Can you work these out from the model? Positions are in its coordinate system, mm. Coordinates: 2 decimals unless noted, no trailing zeros. Loops run counter-clockwise (first coordinate to the right, second up) from the corner with the lowest first, then second, coordinate; pieces in that order, holes last. Notation, with made-up numbers: (29.5, 64) -> (50.5, 64) arc R25 ccw to (50.5, 86) -> close; hole circle Ø10 at (74.5, 65). An arc over 180 degrees is marked (long way). Put each result on its own line as item: value. Start each with the question number.
Item 1: Will this pin go through, and if not, where does the flat tip stop? P1, Ø2.5, axis at x = -91.5, y = -22.5, coming from the +Z side.
Item 2: If we section it at A-A on y = 0: Please give me the cut outline in (x, z), plus the area to 3 significant figures.
Item 3: We'd pull the mould along X, two halves only. Please class faces 1 (the flat face through (-1, 1, 0)), 2 (the cylindrical face through (12.1, -1.2, 1.5)), 3 (the cylindrical face through (-103.08, 35.16, 1.52)): pulls with the +X half, pulls with the -X half, needs draft (parallel to the pull), parting line crosses it, or undercut.
Item 4: Please list where these lines run through material, in increasing order: L1, parallel to Y at x = 102.5, z = 0.85; L2, parallel to Y at x = 10.5, z = 2; L3, parallel to X at y = 1.5, z = 1.6. Write a range as from..to.
```python
from build123d import *

# Parameters (mm, degrees)
SKETCH1_W           = 213
SKETCH1_H           = 77.54
BOSS_EXTRUDE1_DEPTH = 3
FILLET2_R           = 12
CUT_EXTRUDE1_REACH  = 115.377
SKETCH2_R           = 2
CUT_EXTRUDE2_REACH  = 115.377
SKETCH3_R           = 1.5
CUT_EXTRUDE3_REACH  = 115.377
SKETCH4_R           = 1.5


with BuildPart() as part:
    # Sketch1 → Boss-Extrude1 (new body)
    with BuildSketch(Plane.XY):
        Rectangle(SKETCH1_W, SKETCH1_H)
    extrude(amount=BOSS_EXTRUDE1_DEPTH)

    # Fillet2
    fillet2_edges = [part.edges().sort_by_distance(p)[0] for p in [
        (-106.5, 38.77, 1.5),
    ]]
    fillet(fillet2_edges, radius=FILLET2_R)

    # Sketch2 → Cut-Extrude1 (cut, up to next)
    with BuildSketch(Plane(origin=(0, 0, 0), x_dir=(-1, 0, 0), z_dir=(0, 0, -1)), mode=Mode.PRIVATE) as cut_extrude1_sk1:
        with Locations((-10.5, 0)):
            Circle(SKETCH2_R)
    cut_extrude1_tool1 = extrude(cut_extrude1_sk1.sketch, amount=-CUT_EXTRUDE1_REACH, mode=Mode.PRIVATE) & part.part
    add(cut_extrude1_tool1.solids().sort_by_distance((10.5, 0, 0))[0], mode=Mode.SUBTRACT)

    # Sketch3 → Cut-Extrude2 (cut, up to next)
    with BuildSketch(Plane(origin=(0, 0, 0), x_dir=(-1, 0, 0), z_dir=(0, 0, -1)), mode=Mode.PRIVATE) as cut_extrude2_sk1:
        with Locations((-102.5, 22.5)):
            Circle(SKETCH3_R)
    cut_extrude2_tool1 = extrude(cut_extrude2_sk1.sketch, amount=-CUT_EXTRUDE2_REACH, mode=Mode.PRIVATE) & part.part
    # Sketch3 → Cut-Extrude2 (cut, up to next)
    with BuildSketch(Plane(origin=(0, 0, 0), x_dir=(-1, 0, 0), z_dir=(0, 0, -1)), mode=Mode.PRIVATE) as cut_extrude2_sk2:
        with Locations((-102.5, -22.5)):
            Circle(SKETCH3_R)
    cut_extrude2_tool2 = extrude(cut_extrude2_sk2.sketch, amount=-CUT_EXTRUDE2_REACH, mode=Mode.PRIVATE) & part.part
    add(cut_extrude2_tool1.solids().sort_by_distance((102.5, 22.5, 0))[0], mode=Mode.SUBTRACT)
    add(cut_extrude2_tool2.solids().sort_by_distance((102.5, -22.5, 0))[0], mode=Mode.SUBTRACT)

    # Sketch4 → Cut-Extrude3 (cut, up to next)
    with BuildSketch(Plane(origin=(0, 0, 0), x_dir=(-1, 0, 0), z_dir=(0, 0, -1)), mode=Mode.PRIVATE) as cut_extrude3_sk1:
        with Locations((91.5, 22.5)):
            Circle(SKETCH4_R)
    cut_extrude3_tool1 = extrude(cut_extrude3_sk1.sketch, amount=-CUT_EXTRUDE3_REACH, mode=Mode.PRIVATE) & part.part
    # Sketch4 → Cut-Extrude3 (cut, up to next)
    with BuildSketch(Plane(origin=(0, 0, 0), x_dir=(-1, 0, 0), z_dir=(0, 0, -1)), mode=Mode.PRIVATE) as cut_extrude3_sk2:
        with Locations((91.5, -22.5)):
            Circle(SKETCH4_R)
    cut_extrude3_tool2 = extrude(cut_extrude3_sk2.sketch, amount=-CUT_EXTRUDE3_REACH, mode=Mode.PRIVATE) & part.part
    add(cut_extrude3_tool1.solids().sort_by_distance((-91.5, 22.5, 0))[0], mode=Mode.SUBTRACT)
    add(cut_extrude3_tool2.solids().sort_by_distance((-91.5, -22.5, 0))[0], mode=Mode.SUBTRACT)


solid = part.part
```
Solutions:
1. P1: through
2. outline: (-106.5, 0) -> (8.5, 0) -> (8.5, 3) -> (-106.5, 3) -> close; (12.5, 0) -> (106.5, 0) -> (106.5, 3) -> (12.5, 3) -> close
2. area: 627 mm^2
3. face 1: needs draft
3. face 2: undercut
3. face 3: pulls with the -X half
4. L1: -38.77..-24, -21..21, 24..38.77
4. L2: -38.77..-2, 2..38.77
4. L3: -106.5..9.18, 11.82..106.5
